Design review of the part shown in the three views and the two pictorial views. Dimensions are in mm from the part's minimum x, y and z. Round coordinates to 2 decimals unless told otherwise and drop trailing zeros. Write each loop counter-clockwise with the first axis right and the second up, starting at its lowest first coordinate (ties: lowest second). Pieces come first, ordered by that corner, then holes. Notation, with made-up numbers: (60, -15.5) -> (71, -15.5) arc R29 cw to (71, 14.5) -> close; hole circle Ø10 at (-20.5, -14). An arc over 180 degrees is marked (long way). One line per question, with ' | ' between items. Start each with the question number.
1) Consider section B-B (x = 86.5). Give the boundary of the cut face in (y, z).
2) Consider section C-C (z = 2.5). Give the boundary of the cut face in (x, y), then the cut area to 3 significant figures.
3) Insertion check: pin 1 Ø5 at (y, z) = (4, 13) entering from +X (1 decimal); pin 2 Ø3.5 at (x, z) = (3, 12) entering from -Y; pin 3 Ø4 at (y, z) = (3, 10.5) entering from -X. Each pin has a flat end and moves straight along its axis. Give the tip position at first contact, or say it passes through.
4) Consider section A-A (y = 3). Give the boundary of the cut face in (x, z) (1 decimal).
5) For probe 1 along X at (y, z) = (5.25, 2); probe 2 along X at (y, z) = (4.5, 10) (1 decimal); probe 3 along Z at (x, y) = (76.5, 6), list the stretches that pass through material, from the lowest coordinate up.
6) Mouldability with a two-part tool opening along X and no side actions: class the marked faces 1, 2 and 3 as +X half, -X half, draft (parallel to the pull), parting line (faces both ways), or undercut.
7) Consider section D-D (x = 41.5). Give the boundary of the cut face in (y, z).
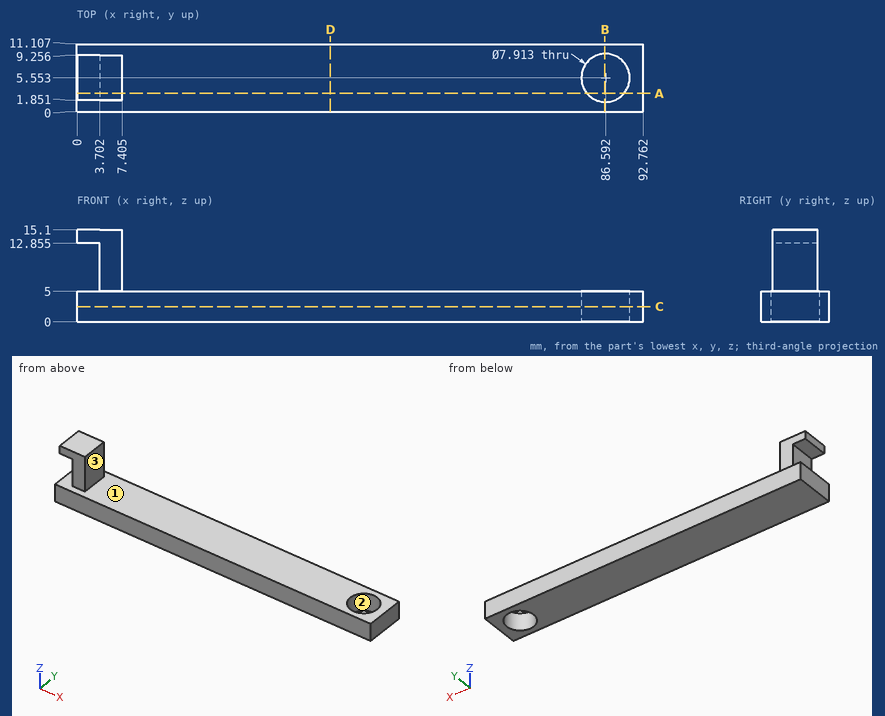
From the geometry:
1) outline: (0, 0) -> (1.6, 0) -> (1.6, 5) -> (0, 5) -> close; (9.51, 0) -> (11.11, 0) -> (11.11, 5) -> (9.51, 5) -> close
2) outline: (0, 0) -> (92.76, 0) -> (92.76, 11.11) -> (0, 11.11) -> close; hole circle Ø7.91 at (86.59, 5.55) | area: 981 mm2
3) pin 1: stops at x = 7.4 | pin 2: stops at y = 1.85 | pin 3: stops at x = 3.7
4) outline: (0, 0) -> (83.6, 0) -> (83.6, 5) -> (7.4, 5) -> (7.4, 15.1) -> (0, 15.1) -> (0, 12.9) -> (3.7, 12.9) -> (3.7, 5) -> (0, 5) -> close; (89.6, 0) -> (92.8, 0) -> (92.8, 5) -> (89.6, 5) -> close
5) probe 1: x = 0 to 82.65, 90.54 to 92.76 | probe 2: x = 3.7 to 7.4 | probe 3: z = 0 to 5
6) face 1: draft | face 2: undercut | face 3: +X half
7) outline: (0, 0) -> (11.11, 0) -> (11.11, 5) -> (0, 5) -> close
